from build123d import *

# Parameters (mm, degrees)
PAD001_DEPTH    = 5
SKETCH014_R     = 1.6
SKETCH014_R_2   = 3.2
POCKET003_DEPTH = 5.001
SKETCH015_R     = 2.85
POCKET004_DEPTH = 3
FILLET001_R     = 4
CHAMFER_SIZE    = 1


with BuildPart() as part:
    # Sketch010 → Pad001 (new body)
    with BuildSketch(Plane.XY):
        with BuildLine():
            Line((44.86111, -50), (59.975919, -16.416677))
            ThreePointArc((59.975919, -16.416677), (62.609058, -8.395333), (63.5, 0))
            Line((57.7, 0), (63.5, 0))
            ThreePointArc((51.3, 0), (54.5, -3.2), (57.7, 0))
            Line((0, 0), (51.3, 0))
            Line((0, -53.373162), (0, 0))
            ThreePointArc((0, -53.373162), (22.493874, -52.528683), (44.86111, -50))
        make_face()
    extrude(amount=-PAD001_DEPTH)

    # Sketch014 (on Face9 of Pad001) → Pocket003 (cut, through all)
    with BuildSketch(Plane(origin=(0, 0, -5), x_dir=(1, 0, 0), z_dir=(0, 0, -1))):
        with Locations((45, 40)):
            Circle(SKETCH014_R)
        with Locations((54.5, 0)):
            Circle(SKETCH014_R_2)
    extrude(amount=-POCKET003_DEPTH, mode=Mode.SUBTRACT)

    # Sketch015 (on Face5 of Pocket003) → Pocket004 (cut)
    with BuildSketch(Plane(origin=(0, 0, -5), x_dir=(1, 0, 0), z_dir=(0, 0, -1))):
        with Locations((45, 40)):
            Circle(SKETCH015_R)
    extrude(amount=-POCKET004_DEPTH, mode=Mode.SUBTRACT)

    # Fillet001
    fillet001_edges = [part.edges().sort_by_distance(p)[0] for p in [
        (44.86111, -50, -2.5),
    ]]
    fillet(fillet001_edges, radius=FILLET001_R)

    # Chamfer
    chamfer_edges = [part.edges().sort_by_distance(p)[0] for p in [
        (21.394971, -52.609282, -5),
    ]]
    chamfer(chamfer_edges, length=CHAMFER_SIZE)


solid = part.part
Geometry check sheet. Reference: the model listing, model coordinates, mm. A direction names the side the tool comes from. Round coordinates to 2 decimals unless told otherwise and drop trailing zeros. Order: outer loops, then holes, each group sorted by start corner. A loop starts at its lowest first (then second) coordinate and runs counter-clockwise, first axis right, second up. Notation, with made-up numbers: M 67.5,0.5 L 116.5,0.5 A32 cw 116.5,39.5 Z; hole C -37,63 d4. An arc over 180 degrees is marked long. Answer in a Markdown table with one row per item.
(1) Scan lines: probe 1 along X at (y, z) = (-40, -2.85); probe 2 along Y at (x, z) = (45, -3.9); probe 3 along Y at (x, z) = (45, -0.45). Record each from-to range of solid material in increasing order. Write a range as from..to.
Responses:
| item | result |
|---|---|
| probe 1 | x = 0..42.15, 47.85..49.36 |
| probe 2 | y = -49.13..-42.85, -37.15..0 |
| probe 3 | y = -49.13..-41.6, -38.4..0 |
(2) Go/stop test with flat-tipped pins: P1, Ø3, axis at x = 7, z = -2.5, coming from the -Y side; P2, Ø1, axis at y = -46, z = -4.5, coming from the +X side; P3, Ø1.5, axis at y = -15.5, z = -2.5, coming from the +X side; P4, Ø3, axis at x = 45, y = -40, coming from the +Z side. Record where each tip stops, or that it passes through.
Responses:
| item | result |
|---|---|
| P1 | stops at y = -53.32 |
| P2 | stops at x = 46.71 |
| P3 | stops at x = 60.68 |
| P4 | passes through |
(3) Sectioned sample at A-A, the plane z = -1.2. Record the cut outline in (x, y).
Responses:
| item | result |
|---|---|
| outline | M 0,-53.37 A300 ccw 42.68,-50.32 A4 ccw 45.76,-48 L 59.98,-16.42 A40 ccw 63.5,0 L 57.7,0 A3.2 cw 51.3,0 L 0,0 Z; hole C 45,-40 d3.2 |
(4) Sectioned sample at C-C, the plane x = 50. Record the cut outline in (y, z).
Responses:
| item | result |
|---|---|
| outline | M -38.58,-4 L -36.15,-5 L 0,-5 L 0,0 L -38.58,0 Z |
(5) Sectioned sample at B-B, the plane y = -40. Record the cut outline in (x, z), and give its area (3 significant figures).
Responses:
| item | result |
|---|---|
| outline | M 0,-5 L 42.15,-5 L 42.15,-2 L 43.4,-2 L 43.4,0 L 0,0 Z; M 46.6,-2 L 47.85,-2 L 47.85,-5 L 48.27,-5 L 49.36,-4 L 49.36,0 L 46.6,0 Z |
| area | 223 mm² |
(6) Sectioned sample at D-D, the plane y = -28. Record the cut outline in (x, z), and give its area (3 significant figures).
Responses:
| item | result |
|---|---|
| outline | M 0,-5 L 53.67,-5 L 54.76,-4 L 54.76,0 L 0,0 Z |
| area | 273 mm² |
(7) Draft check along X on faces 3 (the face through (54.4, -3.2, -2.5)), 4 (the face through (0, -27, -2)), 5 (the face through (24, -26, -5)). Enter one of: released by +X, released by -X, zero draft, split by the parting line, or undercut.
Responses:
| item | result |
|---|---|
| face 3 | undercut |
| face 4 | released by -X |
| face 5 | zero draft |
(8) Tool access check on faces 1 (the face through (25, 0, -2)), 2 (the face through (47, -40, -2)). Record the directions out of +Z, -Z, +X, -X, +Y, -Y that give a thin tool (end or side, any length) a straight path to the whole face; none if there is none.
Responses:
| item | result |
|---|---|
| face 1 | +Z, -Z, +X, -X, +Y |
| face 2 | -Z |
